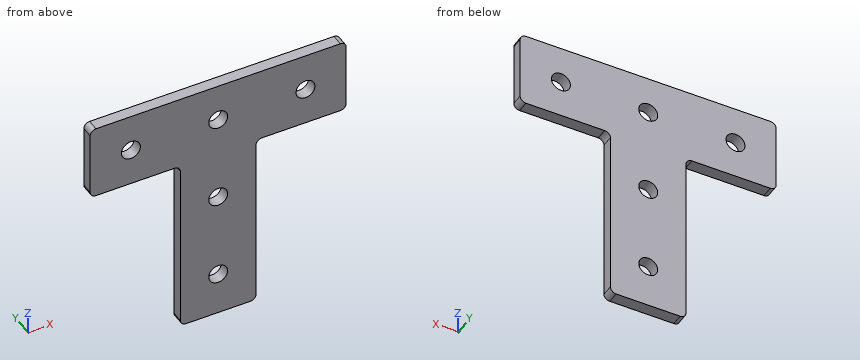
```python
from build123d import *

# Parameters (mm, degrees)
BOSS_EXTRUDE1_DEPTH = 4
SKETCH3_R           = 3.25
CUT_EXTRUDE1_DEPTH  = 88.045964869
FILLET1_R           = 2


with BuildPart() as part:
    # Sketch1 → Boss-Extrude1 (new body)
    with BuildSketch(Plane(origin=(0, 0, 0), x_dir=(1, 0, 0), z_dir=(0, 1, 0))):
        Polygon((-44, 13), (-44, -13), (44, -13), (44, 13), (13, 13), (13, 75), (-13, 75), (-13, 13), align=None)
    extrude(amount=BOSS_EXTRUDE1_DEPTH)

    # Sketch3 → Cut-Extrude1 (cut, through all)
    with BuildSketch(Plane(origin=(0, 4, 0), x_dir=(1, 0, 0), z_dir=(0, 1, 0))):
        with Locations(Location((0, 0, 0), (0, 0, 270))):
            Circle(SKETCH3_R)
        with Locations(Location((30, 0, 0), (0, 0, 270))):
            Circle(SKETCH3_R)
        with Locations(Location((-30, 0, 0), (0, 0, 270))):
            Circle(SKETCH3_R)
        with Locations(Location((0, 60, 0), (0, 0, 270))):
            Circle(SKETCH3_R)
        with Locations(Location((0, 30, 0), (0, 0, 270))):
            Circle(SKETCH3_R)
    extrude(amount=-CUT_EXTRUDE1_DEPTH, mode=Mode.SUBTRACT)

    # Fillet1
    fillet1_edges = [part.edges().sort_by_distance(p)[0] for p in [
        (44, 2, 13),
        (-44, 2, 13),
        (-44, 2, -13),
        (-13, 2, -13),
        (-13, 2, -75),
        (13, 2, -75),
        (13, 2, -13),
        (44, 2, -13),
    ]]
    fillet(fillet1_edges, radius=FILLET1_R)


solid = part.part
```
Read the model definition and answer for the solid it produces. Units are mm, in the model's axes. Give positions to 0.01 mm unless a question says otherwise; leave off trailing zeros. Order: outer loops, then holes, each group sorted by start corner. A loop starts at its lowest first (then second) coordinate and runs counter-clockwise, first axis right, second up. Notation, with made-up numbers: (68.5, 88.25) -> (120.5, 88.25) arc R19 cw to (120.5, 118.25) -> close; hole circle Ø4 at (62.5, -14.75). An arc over 180 degrees is marked (long way). Write item = value, one per line.
1. A cutting plane is placed at C-C, the plane x = 0. Write down the section's boundary in (y, z), and give its area (3 significant figures).
Numbers:
outline = (0, -75) -> (4, -75) -> (4, -63.25) -> (0, -63.25) -> close; (0, -56.75) -> (4, -56.75) -> (4, -33.25) -> (0, -33.25) -> close; (0, -26.75) -> (4, -26.75) -> (4, -3.25) -> (0, -3.25) -> close; (0, 3.25) -> (4, 3.25) -> (4, 13) -> (0, 13) -> close
area = 274 mm²
2. A cutting plane is placed at B-B, the plane z = -60. Write down the section's boundary in (x, y).
Numbers:
outline = (-13, 0) -> (-3.25, 0) -> (-3.25, 4) -> (-13, 4) -> close; (3.25, 0) -> (13, 0) -> (13, 4) -> (3.25, 4) -> close
3. A cutting plane is placed at A-A, the plane x = 30. Write down the section's boundary in (y, z).
Numbers:
outline = (0, -13) -> (4, -13) -> (4, -3.25) -> (0, -3.25) -> close; (0, 3.25) -> (4, 3.25) -> (4, 13) -> (0, 13) -> close
4. A cutting plane is placed at D-D, the plane y = 1.5. Write down the section's boundary in (x, z), and give its area (3 significant figures).
Numbers:
outline = (-44, -11) arc R2 ccw to (-42, -13) -> (-15, -13) arc R2 cw to (-13, -15) -> (-13, -73) arc R2 ccw to (-11, -75) -> (11, -75) arc R2 ccw to (13, -73) -> (13, -15) arc R2 cw to (15, -13) -> (42, -13) arc R2 ccw to (44, -11) -> (44, 11) arc R2 ccw to (42, 13) -> (-42, 13) arc R2 ccw to (-44, 11) -> close; hole circle Ø6.5 at (-30, 0); hole circle Ø6.5 at (0, -60); hole circle Ø6.5 at (0, -30); hole circle Ø6.5 at (0, 0); hole circle Ø6.5 at (30, 0)
area = 3,730 mm²
5. Given pin 1 (1.2 mm diameter, centred on y = 1.5, z = -47.5, fed in from +X); pin 2 (5 mm diameter, centred on x = 0, z = 0, fed in from -Y); pin 3 (1.2 mm diameter, centred on x = 32, y = 2, fed in from -Z), each flat-ended and moving along its own axis, determine where each tip first touches the part or whether it passes through.
Numbers:
pin_1 = 13
pin_2 = through
pin_3 = -13
6. Straight lines are drawn through the part: line 1 along X through (y, z) = (2.8, 0); line 2 along X through (y, z) = (2.2, -30); line 3 along X through (y, z) = (2.45, -1). For each, find the intervals that lie inside material, in ascending order.
Numbers:
line_1 = -44 to -33.25, -26.75 to -3.25, 3.25 to 26.75, 33.25 to 44
line_2 = -13 to -3.25, 3.25 to 13
line_3 = -44 to -33.09, -26.91 to -3.09, 3.09 to 26.91, 33.09 to 44
